Design review of the part built by this model. Coordinates are the model's own, in mm. Face numbers are marked on the shaded views. Give positions to 0.01 mm unless a question says otherwise; leave off trailing zeros. Write each loop counter-clockwise with the first axis right and the second up, starting at its lowest first coordinate (ties: lowest second). Pieces come first, ordered by that corner, then holes. Notation, with made-up numbers: M -17,-29.75 L 21,-29.75 A24 ccw 21,-11.75 Z; hole C 29,44.25 d1. An arc over 180 degrees is marked long. One line per item, written item: value. Start each with the question number.
```python
from build123d import *

# Parameters (mm, degrees)
F6_DEPTH = 9.501


# Not quite as in the source:
# - a feature of the source that left no trace in its solid (it failed there, or was rolled back) is left out
# - the program builds the solid bodies; features that only make, move or delete a surface that nothing else refers to are left out


with BuildPart() as f4:
    # F0 (on Top) → F4 (revolve)
    with BuildSketch(Plane.XY):
        Polygon((34.4624469289, 70.1398981537), (36.5624469289, 70.1398981537), (36.5624469289, 75.9898981537), (20.4008240253, 75.9898981537), (20.4008240253, 66.4898981537), (28.4008240253, 66.4898981537), (34.4624469289, 66.4898981537), align=None)
    revolve(axis=Axis((47.0624469289, 47.4898981537, 0), (0, -1, 0)))

    # F5 (on face) → F6 (cut, through all)
    with BuildSketch(Plane(origin=(0, 75.9898981537, 0), x_dir=(-1, 0, 0), z_dir=(0, 1, 0))):
        with BuildLine():
            Line((-53.2110722647, 8.511427993), (-53.2110722647, 25.9429478343))
            ThreePointArc((-53.2110722647, 25.9429478343), (-73.7240698325, 0), (-53.2110722647, -25.9429478343))
            Line((-53.2110722647, -25.9429478343), (-53.2110722647, -8.511427993))
            ThreePointArc((-53.2110722647, -8.511427993), (-57.5624469289, 0), (-53.2110722647, 8.511427993))
        make_face()
    extrude(amount=-F6_DEPTH, mode=Mode.SUBTRACT)


solid = f4.part
```
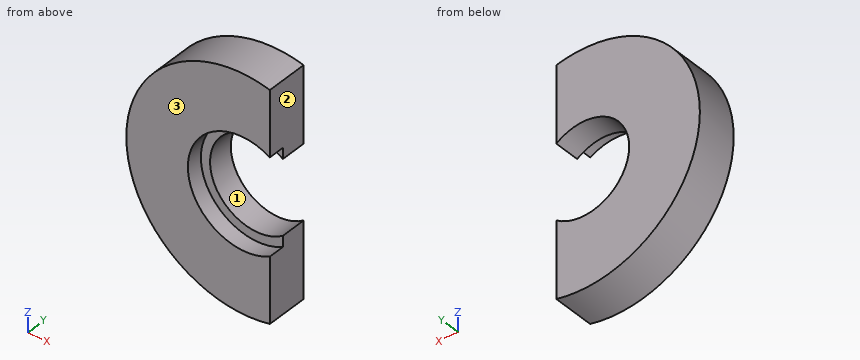
Q1. For P1, Ø4, axis at x = 28, y = 73.5, coming from the -Z side; P2, Ø1, axis at x = 30.5, y = 70, coming from the -Z side; P3, Ø4, axis at y = 69.5, z = -3.5, coming from the +X side, all flat-tipped, find the tip position at first contact; note any pin that passes through.
Q2. The part is to be moulded in two halves that separate along X. For the marked faces 1, 2 and 3, say which applies: pulls with the +X half, pulls with the -X half, needs draft (parallel to the pull), parting line crosses it, or undercut.
Q3. Take a section at A-A, the plane x = 50.5. Give the boundary of the cut face in (y, z).
Q4. Take a section at B-B, the plane z = 0. Give the boundary of the cut face in (x, y), then the cut area to 3 significant figures.
Q5. Take a section at D-D, the plane x = 36. Give the boundary of the cut face in (y, z).
Q6. Wall thickness on line 1 (X direction, y = 73.3, z = 0); line 2 (Z direction, x = 52.5, y = 71); line 3 (X direction, y = 73, z = 23.5): over which ranges is each line inside the solid? List them lowest first. Write a range as from..to.
Q7. Take a section at C-C, the plane y = 74.25. Give the boundary of the cut face in (x, z), then the cut area to 3 significant figures.
Results list:
1. P1: stops at z = -20.49
1. P2: stops at z = -21.28
1. P3: stops at x = 38.05
2. face 1: undercut
2. face 2: pulls with the +X half
2. face 3: needs draft
3. outline: M 66.49,-26.44 L 75.99,-26.44 L 75.99,-9.92 L 70.14,-9.92 L 70.14,-12.12 L 66.49,-12.12 Z; M 66.49,12.12 L 70.14,12.12 L 70.14,9.92 L 75.99,9.92 L 75.99,26.44 L 66.49,26.44 Z
4. outline: M 20.4,66.49 L 34.46,66.49 L 34.46,70.14 L 36.56,70.14 L 36.56,75.99 L 20.4,75.99 Z
4. area: 146 mm^2
5. outline: M 66.49,-24.26 L 75.99,-24.26 L 75.99,24.26 L 66.49,24.26 L 66.49,6.03 L 70.14,6.03 L 70.14,-6.03 L 66.49,-6.03 Z
6. line 1: x = 20.4..36.56
6. line 2: z = -26.1..-8.98, 8.98..26.1
6. line 3: x = 34.47..53.21
7. outline: M 53.21,-25.94 L 53.21,-8.51 A10.5 cw long 53.21,8.51 L 53.21,25.94 A26.66 ccw long Z
7. area: 1,150 mm^2
